Geometry: final body of the model. Coordinates: model frame, mm. A direction names the side the tool comes from. Round coordinates to 2 decimals unless told otherwise and drop trailing zeros. Loops run counter-clockwise (first coordinate to the right, second up) from the corner with the lowest first, then second, coordinate; pieces in that order, holes last. Notation, with made-up numbers: (26.25, 77) -> (71.25, 77) arc R32 cw to (71.25, 115) -> close; hole circle Ø2 at (62, -19.75). An arc over 180 degrees is marked (long way). Answer in a Markdown table with one row per item.
```python
from build123d import *

# Parameters (mm, degrees)
CUT_EXTRUDE_1_DEPTH = 2.5
FILLET_1_R          = 0.3
CHAMFER_1_SIZE      = 1


with BuildPart() as part:
    # Эскиз1 → Повернуть1 (revolve)
    with BuildSketch(Plane.XY):
        Polygon((0, 0), (0, 5), (6, 5), (6, 3), (46, 3), (46, 0), align=None)
    revolve(axis=Axis((46, 0, 0), (-1, 0, 0)))

    # Эскиз2 → Вырез-Вытянуть1 (cut)
    with BuildSketch(Plane.ZY):
        Polygon((-1.443375673, 2.5), (-2.886751346, 0), (-1.443375673, -2.5), (1.443375673, -2.5), (2.886751346, 0), (1.443375673, 2.5), align=None)
    extrude(amount=-CUT_EXTRUDE_1_DEPTH, mode=Mode.SUBTRACT)

    # Скругление1
    fillet_1_edges = [part.edges().sort_by_distance(p)[0] for p in [
        (6, -3, 0),
        (0, -5, 0),
    ]]
    fillet(fillet_1_edges, radius=FILLET_1_R)

    # Фаска1
    chamfer_1_edges = [part.edges().sort_by_distance(p)[0] for p in [
        (46, -3, 0),
    ]]
    chamfer(chamfer_1_edges, length=CHAMFER_1_SIZE)


solid = part.part
```
Item 1: Cut plane B-B (x = 12). Output: boundary loops of the cut face in (y, z).
Answer:
| item | result |
|---|---|
| outline | circle Ø6 at (0, 0) |
Item 2: Draft query along Y for faces 4 (the face through (1.232, -1.267, 2.155)), 5 (the face through (26, -3, 0)), 6 (the face through (46, 0, 0)). Return one class per face: pulls with the +Y half, pulls with the -Y half, needs draft (parallel to the pull), parting line crosses it, or undercut.
Answer:
| item | result |
|---|---|
| face 4 | undercut |
| face 5 | parting line crosses it |
| face 6 | needs draft |
Item 3: Cut plane A-A (z = 0). Output: boundary loops of the cut face in (x, y).
Answer:
| item | result |
|---|---|
| outline | (0, -4.7) arc R0.3 ccw to (0.3, -5) -> (6, -5) -> (6, -3.3) arc R0.3 cw to (6.3, -3) -> (45, -3) -> (46, -2) -> (46, 2) -> (45, 3) -> (6.3, 3) arc R0.3 cw to (6, 3.3) -> (6, 5) -> (0.3, 5) arc R0.3 ccw to (0, 4.7) -> (0, 2.5) -> (2.5, 2.5) -> (2.5, -2.5) -> (0, -2.5) -> close |
Item 4: Pin query (flat end, axial travel): pin 1 Ø1 at (x, y) = (19, 1) entering from +Z; pin 2 Ø1.5 at (x, y) = (16.5, -2) entering from +Z; pin 3 Ø2 at (x, y) = (20.5, -3.5) entering from +Z. Return the tip coordinate at first contact, or that it passes through.
Answer:
| item | result |
|---|---|
| pin 1 | stops at z = 2.96 |
| pin 2 | stops at z = 2.73 |
| pin 3 | stops at z = 1.66 |
Item 5: Reachability of faces 1 (the face through (1.232, 1.267, -2.155)), 2 (the face through (6, 3.3, -1.2)), 3 (the face through (0, -2, 2)) from +Z, -Z, +X, -X, +Y, -Y: full face, straight path, thin tool, end or side. Return the list, or none.
Answer:
| item | result |
|---|---|
| face 1 | -X |
| face 2 | +X |
| face 3 | +Z, -Z, -X, +Y, -Y |
Item 6: Line query: probe 1 along X at (y, z) = (-4.25, 1.5); probe 2 along Z at (x, y) = (10, 0); probe 3 along X at (y, z) = (0.5, -1.5). Output: solid intervals per line, ascending. Write a range as [from, to].
Answer:
| item | result |
|---|---|
| probe 1 | x = [0, 6] |
| probe 2 | z = [-3, 3] |
| probe 3 | x = [2.5, 46] |
